```python
from build123d import *

# Parameters (mm, degrees)
SKETCH1_W           = 9
SKETCH1_H           = 9
BOSS_EXTRUDE1_DEPTH = 3
HOLE1_D             = 4
HOLE1_CBORE_D       = 5
HOLE1_CBORE_DEPTH   = 0.8
BOSS_EXTRUDE3_DEPTH = 2.2
HOLE2_D             = 4
HOLE2_DEPTH         = 2.2
HOLE2_CBORE_D       = 5
HOLE2_CBORE_DEPTH   = 0.8
SKETCH7_R           = 2.5
CUT_EXTRUDE1_DEPTH  = 0.8
SKETCH8_R           = 2.5
CUT_EXTRUDE2_DEPTH  = 0.8


with BuildPart() as part:
    # Sketch1 → Boss-Extrude1 (new body)
    with BuildSketch(Plane.XY):
        with Locations((-4.5, 4.5)):
            Rectangle(SKETCH1_W, SKETCH1_H)
    extrude(amount=BOSS_EXTRUDE1_DEPTH)

    # Hole1 (through all)
    with Locations(Plane.XY.offset(3)):
        with Locations((0, 0), (-6, 0), (0, 6)):
            CounterBoreHole(HOLE1_D / 2, HOLE1_CBORE_D / 2, HOLE1_CBORE_DEPTH)

    # Sketch4 → Boss-Extrude3 (add)
    with BuildSketch(Plane.ZY.offset(9)):
        with BuildLine():
            Line((0, 9), (0, 3))
            ThreePointArc((0, 3), (-3, 6), (0, 9))
        make_face()
    extrude(amount=-BOSS_EXTRUDE3_DEPTH)

    # Hole2
    with Locations(Plane.ZY.offset(9)):
        with Locations((0, 6)):
            CounterBoreHole(HOLE2_D / 2, HOLE2_CBORE_D / 2, HOLE2_CBORE_DEPTH, depth=HOLE2_DEPTH)

    # Sketch7 → Cut-Extrude1 (cut)
    with BuildSketch(Plane(origin=(0, 0, 0), x_dir=(-1, 0, 0), z_dir=(0, 0, -1))):
        with Locations((0, 6)):
            Circle(SKETCH7_R)
        Circle(SKETCH7_R)
        with Locations((6, 0)):
            Circle(SKETCH7_R)
    extrude(amount=-CUT_EXTRUDE1_DEPTH, mode=Mode.SUBTRACT)

    # Sketch8 → Cut-Extrude2 (cut)
    with BuildSketch(Plane(origin=(-6.8, 0, 0), x_dir=(0, 0, -1), z_dir=(1, 0, 0))):
        with Locations((0, 6)):
            Circle(SKETCH8_R)
    extrude(amount=CUT_EXTRUDE2_DEPTH, mode=Mode.SUBTRACT)

    # Mirror1: part across plane


with BuildPart() as part_1:
    add(part.part)
    add(part.part.mirror(Plane(origin=(0, 0, 0), x_dir=(0, 0, 1), z_dir=(1, 0, 0))))

    # Mirror2: part across plane


with BuildPart() as part_2:
    add(part_1.part)
    add(part_1.part.mirror(Plane.ZX))


solid = part_2.part
```
Geometry: final body of the model. Coordinates: model frame, mm. A direction names the side the tool comes from. Give positions to 0.01 mm unless a question says otherwise; leave off trailing zeros. Loops run counter-clockwise (first coordinate to the right, second up) from the corner with the lowest first, then second, coordinate; pieces in that order, holes last. Notation, with made-up numbers: (84, 8) -> (126, 8) arc R8 ccw to (126, 23) -> close; hole circle Ø7 at (50, -39). An arc over 180 degrees is marked (long way). Use CSV: the item, a comma, the result in double quotes.
(1) Access query for faces 5 (the face through (-5, -2, 0.8)), 6 (the face through (1, 8, 2.2)), 7 (the face through (-4.4, 1.2, 1.5)). Directions: +Z, -Z, +X, -X, +Y, -Y. A direction counts if a zero-diameter tool reaches every point of the face in a straight line with its end or side. Return the directions, or none.
From the geometry:
face 5,"-Z"
face 6,"+Z"
face 7,"+Z, -Z"
(2) Cut plane B-B (y = 6). Count the separate pieces of the cut face and the enclosed holes in it, plus the area to 3 significant figures.
From the geometry:
separate pieces,"4"
enclosed holes,"0"
area,"30.4 mm^2"
(3) Pull-direction query (Z, two-part tool) for faces 1 (the face through (-8, -6, -3)), 2 (the face through (-7, -2, 2.2)), 3 (the face through (8.61, -8.48, -0.33)), 4 (the face through (-8.2, 8, -1)); classes: released by +Z, released by -Z, zero draft, split by the parting line, or undercut.
From the geometry:
face 1,"released by -Z"
face 2,"released by +Z"
face 3,"undercut"
face 4,"undercut"
(4) Ray query, line 1 along Y through (x, z) = (1.5, 0.4); line 2 along Y through (x, z) = (-7.75, 0.9); line 3 along Z through (x, y) = (-5, 3). Return the intervals inside material, ascending. Write a range as [from, to].
From the geometry:
line 1,"[-9, -8], [-4, -2], [2, 4], [8, 9]"
line 2,"[-9, -7.79], [-4.21, -0.97], [0.97, 4.21], [7.79, 9]"
line 3,"[0, 3]"
(5) Cut plane C-C (y = 8.25). Output: boundary loops of the cut face in (x, z), plus the area to 3 significant figures.
From the geometry:
outline,"(-9, -1.98) -> (-6.8, -1.98) -> (-6.8, 1.09) -> (-6, 1.09) -> (-6, 0) -> (-1.09, 0) -> (-1.09, 0.8) -> (1.09, 0.8) -> (1.09, 0) -> (6, 0) -> (6, 1.09) -> (6.8, 1.09) -> (6.8, -1.98) -> (9, -1.98) -> (9, -1.09) -> (8.2, -1.09) -> (8.2, 1.09) -> (9, 1.09) -> (9, 3) -> (1.09, 3) -> (1.09, 2.2) -> (-1.09, 2.2) -> (-1.09, 3) -> (-9, 3) -> (-9, 1.09) -> (-8.2, 1.09) -> (-8.2, -1.09) -> (-9, -1.09) -> close"
area,"54.0 mm^2"
(6) Cut plane A-A (x = 5). Output: boundary loops of the cut face in (y, z), plus the area to 3 significant figures.
From the geometry:
outline,"(-9, 0) -> (-2.29, 0) -> (-2.29, 0.8) -> (-1.73, 0.8) -> (-1.73, 2.2) -> (-2.29, 2.2) -> (-2.29, 3) -> (-9, 3) -> close; (1.73, 0.8) -> (2.29, 0.8) -> (2.29, 0) -> (9, 0) -> (9, 3) -> (2.29, 3) -> (2.29, 2.2) -> (1.73, 2.2) -> close"
area,"41.8 mm^2"
(7) First-contact query: P1, Ø1.2, axis at y = -6.5, z = 1.5, coming from the -X side; P2, Ø6, axis at x = 0, y = 6, coming from the -Z side; P3, Ø2, axis at x = 6, z = -0.5, coming from the -Y side. Flat tips, straight axial feed; report the tip coordinate or a pass-through.
From the geometry:
P1,"x = -8.2"
P2,"z = 0"
P3,"y = -9"
